Geometry check sheet. Reference: the model listing, model coordinates, mm. Face numbers are marked on the shaded views. A direction names the side the tool comes from. Coordinates: 2 decimals unless noted, no trailing zeros. Loops run counter-clockwise (first coordinate to the right, second up) from the corner with the lowest first, then second, coordinate; pieces in that order, holes last. Notation, with made-up numbers: (38.5, -35.75) -> (71.5, -35.75) arc R18 ccw to (71.5, -10.75) -> close; hole circle Ø1 at (-1.75, 33). An arc over 180 degrees is marked (long way). Answer as a JSON object with one key per item and string values.
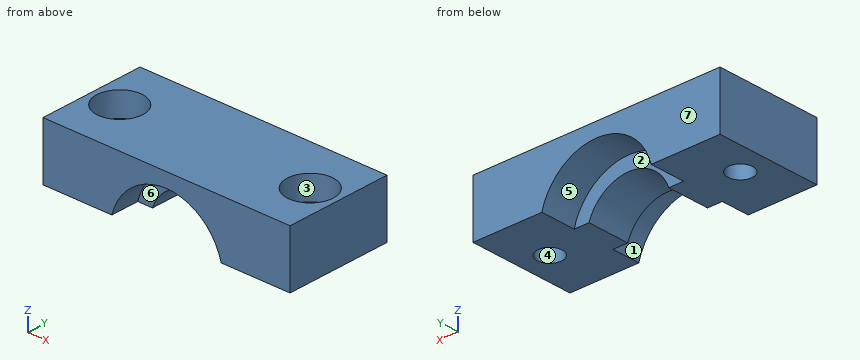
from build123d import *

# Parameters (mm, degrees)
SKETCH1_W                                           = 35
SKETCH1_H                                           = 15
BOSS_EXTRUDE1_DEPTH                                 = 10
CUT_REVOLVE1_ANGLE                                  = 180
SKETCH3_R                                           = 1.75
CUT_EXTRUDE1_DEPTH                                  = 22.505813168
CBORE_FOR_M3_HEX_SOCKET_HEAD_CAP_SCREW1_D           = 3.4
CBORE_FOR_M3_HEX_SOCKET_HEAD_CAP_SCREW1_CBORE_D     = 6.5
CBORE_FOR_M3_HEX_SOCKET_HEAD_CAP_SCREW1_CBORE_DEPTH = 3.4
SKETCH6_W                                           = 35
SKETCH6_H                                           = 4
CUT_EXTRUDE2_DEPTH                                  = 26.124689053


with BuildPart() as part:
    # Sketch1 → Boss-Extrude1 (new body)
    with BuildSketch(Plane.XY):
        Rectangle(SKETCH1_W, SKETCH1_H)
    extrude(amount=BOSS_EXTRUDE1_DEPTH)

    # Sketch2 → Cut-Revolve1 (revolve, cut)
    with BuildSketch(Plane(origin=(0, 0, 0), x_dir=(-1, 0, 0), z_dir=(0, 0, -1))):
        Polygon((0, 7.5), (8, 7.5), (8, 2.5), (6, 2.5), (6, -3.5), (8, -3.5), (8, -7.5), (0, -7.5), align=None)
    revolve(axis=Axis((0, 7.5, 0), (0, 1, 0)), revolution_arc=CUT_REVOLVE1_ANGLE, mode=Mode.SUBTRACT)

    # Sketch3 → Cut-Extrude1 (cut, through all)
    with BuildSketch(Plane.XY.offset(10)):
        with Locations((-13.5, 0)):
            Circle(SKETCH3_R)
        with Locations((13.5, 0)):
            Circle(SKETCH3_R)
    extrude(amount=-CUT_EXTRUDE1_DEPTH, mode=Mode.SUBTRACT)

    # CBORE for M3 Hex Socket Head Cap Screw1 (through all)
    with Locations(Plane.XY.offset(10)):
        with Locations((-13.5, 0), (13.5, 0)):
            CounterBoreHole(CBORE_FOR_M3_HEX_SOCKET_HEAD_CAP_SCREW1_D / 2, CBORE_FOR_M3_HEX_SOCKET_HEAD_CAP_SCREW1_CBORE_D / 2, CBORE_FOR_M3_HEX_SOCKET_HEAD_CAP_SCREW1_CBORE_DEPTH)

    # Sketch6 → Cut-Extrude2 (cut, through all)
    with BuildSketch(Plane(origin=(0, 7.5, 0), x_dir=(1, 0, 0), z_dir=(0, 1, 0))):
        Rectangle(SKETCH6_W, SKETCH6_H)
    extrude(amount=-CUT_EXTRUDE2_DEPTH, mode=Mode.SUBTRACT)


solid = part.part
1. Thickness scan on probe 1 along Y at (x, z) = (-13.5, 5.25); probe 2 along X at (y, z) = (2.25, 6.75); probe 3 along Y at (x, z) = (-13.5, 7.3). Record the ranges inside material, lowest first. Write a range as from..to.
Evaluation:
{"probe 1": "y = -7.5..-1.75, 1.75..7.5", "probe 2": "x = -17.5..-15.85, -11.15..11.15, 15.85..17.5", "probe 3": "y = -7.5..-3.25, 3.25..7.5"}
2. Tool access check on the marked faces 1, 2 and 3. Record the directions out of +Z, -Z, +X, -X, +Y, -Y that give a thin tool (end or side, any length) a straight path to the whole face; none if there is none.
Evaluation:
{"face 1": "-Z, -Y", "face 2": "-Z, +Y", "face 3": "+Z"}
3. Section check A-A, the plane x = -13.5. Record the boundary of the cut face in (y, z).
Evaluation:
{"outline": "(-7.5, 2) -> (-1.75, 2) -> (-1.75, 6.6) -> (-3.25, 6.6) -> (-3.25, 10) -> (-7.5, 10) -> close; (1.75, 2) -> (7.5, 2) -> (7.5, 10) -> (3.25, 10) -> (3.25, 6.6) -> (1.75, 6.6) -> close"}
4. Section check C-C, the plane y = 0. Record the boundary of the cut face in (x, z).
Evaluation:
{"outline": "(-17.5, 2) -> (-15.25, 2) -> (-15.25, 6.6) -> (-16.75, 6.6) -> (-16.75, 10) -> (-17.5, 10) -> close; (-11.75, 2) -> (-5.66, 2) arc R6 cw to (5.66, 2) -> (11.75, 2) -> (11.75, 6.6) -> (10.25, 6.6) -> (10.25, 10) -> (-10.25, 10) -> (-10.25, 6.6) -> (-11.75, 6.6) -> close; (15.25, 2) -> (17.5, 2) -> (17.5, 10) -> (16.75, 10) -> (16.75, 6.6) -> (15.25, 6.6) -> close"}
5. Mould release check, pull along Y, two halves, no side actions. Record for the marked faces 4, 5, 6 and 7: released by +Y, released by -Y, zero draft, split by the parting line, or undercut.
Evaluation:
{"face 4": "undercut", "face 5": "zero draft", "face 6": "released by -Y", "face 7": "released by +Y"}
6. Depth check by flat-ended pin: P1, Ø5, axis at x = -13.5, y = 0, coming from the +Z side; P2, Ø2, axis at x = -1, y = -2, coming from the -Z side; P3, Ø7, axis at x = 15, y = 0, coming from the +Z side; P4, Ø3, axis at x = -3, z = 5, coming from the -Y side. Enter the tip coordinate at first touch or a pass-through.
Evaluation:
{"P1": "stops at z = 6.6", "P2": "stops at z = 5.66", "P3": "stops at z = 10", "P4": "stops at y = -3.5"}
7. Section check B-B, the plane z = 3.5. Record the boundary of the cut face in (x, y).
Evaluation:
{"outline": "(-17.5, -7.5) -> (-7.19, -7.5) -> (-7.19, -3.5) -> (-4.87, -3.5) -> (-4.87, 2.5) -> (-7.19, 2.5) -> (-7.19, 7.5) -> (-17.5, 7.5) -> close; (4.87, -3.5) -> (7.19, -3.5) -> (7.19, -7.5) -> (17.5, -7.5) -> (17.5, 7.5) -> (7.19, 7.5) -> (7.19, 2.5) -> (4.87, 2.5) -> close; hole circle Ø3.5 at (-13.5, 0); hole circle Ø3.5 at (13.5, 0)"}
8. Section check D-D, the plane z = 9. Record the boundary of the cut face in (x, y).
Evaluation:
{"outline": "(-17.5, -7.5) -> (17.5, -7.5) -> (17.5, 7.5) -> (-17.5, 7.5) -> close; hole circle Ø6.5 at (-13.5, 0); hole circle Ø6.5 at (13.5, 0)"}
